The listing builds one solid part. Answer for the finished solid, in the listing's coordinates (mm). A direction names the side the tool comes from. Round coordinates to 2 decimals unless told otherwise and drop trailing zeros. Write each loop counter-clockwise with the first axis right and the second up, starting at its lowest first coordinate (ties: lowest second). Pieces come first, ordered by that corner, then holes. Notation, with made-up numbers: (44.5, -23.5) - (56.5, -23.5) arc R14 cw to (56.5, -12.5) - close; hole circle Ø3 at (84.25, 32.5). An arc over 180 degrees is marked (long way). Answer in a Markdown table with one row per item.
from build123d import *

# Parameters (mm, degrees)
F0_R     = 12.7
F1_DEPTH = 76.2
F2_R     = 6.35
F3_DEPTH = 82.55


with BuildPart() as f1:
    # F0 (on Top) → F1 (new body, symmetric)
    with BuildSketch(Plane.XY):
        Circle(F0_R)
    extrude(amount=F1_DEPTH, both=True)

    # F2 (on Top) → F3 (join, symmetric)
    with BuildSketch(Plane.XY):
        Circle(F2_R)
    extrude(amount=F3_DEPTH, both=True)


solid = f1.part
(1) Find the intervals of material crossed by line 1 (Z direction, x = -10.5, y = -1); line 2 (X direction, y = 0.75, z = -47); line 3 (X direction, y = -3.75, z = 75.5), in increasing order.
Checked values:
| item | result |
|---|---|
| line 1 | z = -76.2 to 76.2 |
| line 2 | x = -12.68 to 12.68 |
| line 3 | x = -12.13 to 12.13 |
(2) For faces 1 (the cylindrical face through (-1.38, -6.2, 79.42)), 2 (the cylindrical face through (-1.38, -6.2, -79.33)), 3 (the flat face through (0, 0, 82.55)), determine the directions among +Z, -Z, +X, -X, +Y, -Y from which every point of the face is accessible in a straight line to the end or side of a thin tool.
Checked values:
| item | result |
|---|---|
| face 1 | +Z |
| face 2 | -Z |
| face 3 | +Z, +X, -X, +Y, -Y |
(3) Section A-A (x = 0) is taken. Give the vertices of the cut face in (y, z), and give its area (3 significant figures).
Checked values:
| item | result |
|---|---|
| outline | (-12.7, -76.2) - (-6.35, -76.2) - (-6.35, -82.55) - (6.35, -82.55) - (6.35, -76.2) - (12.7, -76.2) - (12.7, 76.2) - (6.35, 76.2) - (6.35, 82.55) - (-6.35, 82.55) - (-6.35, 76.2) - (-12.7, 76.2) - close |
| area | 4,030 mm2 |
(4) Flat-ended cylindrical pins translate along their axes: pin 1 (1 mm diameter, centred on y = -3.5, z = -31, fed in from -X); pin 2 (1.5 mm diameter, centred on y = 4.5, z = 36.5, fed in from -X); pin 3 (1.5 mm diameter, centred on y = 8.5, z = 62, fed in from +X). Find the tip coordinate at first contact, or state that the pin passes through.
Checked values:
| item | result |
|---|---|
| pin 1 | stops at x = -12.34 |
| pin 2 | stops at x = -12.13 |
| pin 3 | stops at x = 10.06 |
(5) Section C-C (z = -18) is taken. Give the vertices of the cut face in (x, y), and give its area (3 significant figures).
Checked values:
| item | result |
|---|---|
| outline | circle Ø25.4 at (0, 0) |
| area | 507 mm2 |
(6) Section D-D (y = 9.5) is taken. Give the vertices of the cut face in (x, z), and give its area (3 significant figures).
Checked values:
| item | result |
|---|---|
| outline | (-8.43, -76.2) - (8.43, -76.2) - (8.43, 76.2) - (-8.43, 76.2) - close |
| area | 2,570 mm2 |
